```python
from build123d import *

# Parameters (mm, degrees)
F0_R     = 24
F0_R_2   = 21
F1_DEPTH = 17.5
F3_DEPTH = 12.5


with BuildPart() as f1:
    # F0 (on Front) → F1 (new body, symmetric)
    with BuildSketch(Plane.XZ):
        Circle(F0_R)
        Circle(F0_R_2, mode=Mode.SUBTRACT)
    extrude(amount=F1_DEPTH, both=True)

    # F2 (on Front) → F3 (join, symmetric)
    with BuildSketch(Plane.XZ):
        with BuildLine():
            Line((251.8847116829, -177.5), (236.7270928985, -165.6737260034))
            Line((236.7270928985, -165.6737260034), (28.1491312931, -2.9370746409))
            Line((28.1491312931, -2.9370746409), (23.9981043859, 0.3016386602))
            ThreePointArc((23.9981043859, 0.3016386602), (18.9220383946, -14.7633486375), (5.543918589, -23.350909333))
            Line((5.543918589, -23.350909333), (9.6949454961, -26.5896226342))
            Line((9.6949454961, -26.5896226342), (218.2729071015, -189.3262739966))
            Line((218.2729071015, -189.3262739966), (227.5, -196.5254343899))
            Line((227.5, -196.5254343899), (227.5, -222.5))
            Line((227.5, -222.5), (272.5, -222.5))
            Line((272.5, -222.5), (272.5, -177.5))
            Line((272.5, -177.5), (251.8847116829, -177.5))
        make_face()
        with BuildLine():
            Line((-272.5, -222.5), (-227.5, -222.5))
            Line((-227.5, -222.5), (-227.5, -196.5254343899))
            Line((-227.5, -196.5254343899), (-218.2729071015, -189.3262739966))
            Line((-218.2729071015, -189.3262739966), (-9.6949454961, -26.5896226342))
            Line((-9.6949454961, -26.5896226342), (-5.543918589, -23.350909333))
            ThreePointArc((-5.543918589, -23.350909333), (-18.9220383946, -14.7633486375), (-23.9981043859, 0.3016386602))
            Line((-23.9981043859, 0.3016386602), (-28.1491312931, -2.9370746409))
            Line((-28.1491312931, -2.9370746409), (-236.7270928985, -165.6737260034))
            Line((-236.7270928985, -165.6737260034), (-251.8847116829, -177.5))
            Line((-251.8847116829, -177.5), (-272.5, -177.5))
            Line((-272.5, -177.5), (-272.5, -222.5))
        make_face()
    extrude(amount=F3_DEPTH, both=True)


solid = f1.part
```
Read the model definition and answer for the solid it produces. Units are mm, in the model's axes. A direction names the side the tool comes from. Round coordinates to 2 decimals unless told otherwise and drop trailing zeros. Loops run counter-clockwise (first coordinate to the right, second up) from the corner with the lowest first, then second, coordinate; pieces in that order, holes last. Notation, with made-up numbers: (70.5, 74.5) -> (91.5, 74.5) arc R18 cw to (91.5, 84.5) -> close; hole circle Ø5 at (-37.5, 56). An arc over 180 degrees is marked (long way). One line per item, written item: value.
1) The mould has two halves that part along X. Classify faces 6 (the face through (-227.5, 0, -210)), 7 (the face through (272.5, 0, -200)), 8 (the face through (-0.1, -17.5, -21.2)): pulls with the +X half, pulls with the -X half, needs draft (parallel to the pull), parting line crosses it, or undercut.
Answer list:
face 6: undercut
face 7: pulls with the +X half
face 8: needs draft
2) A cutting plane is placed at C-C (z = -170). Determine the outline of the cut face in (x, y).
Answer list:
outline: (-242.27, -12.5) -> (-193.5, -12.5) -> (-193.5, 12.5) -> (-242.27, 12.5) -> close; (193.5, -12.5) -> (242.27, -12.5) -> (242.27, 12.5) -> (193.5, 12.5) -> close
3) A cutting plane is placed at B-B (y = 0). Determine the outline of the cut face in (x, z).
Answer list:
outline: (-272.5, -222.5) -> (-227.5, -222.5) -> (-227.5, -196.53) -> (-5.54, -23.35) arc R24 ccw to (5.54, -23.35) -> (227.5, -196.53) -> (227.5, -222.5) -> (272.5, -222.5) -> (272.5, -177.5) -> (251.88, -177.5) -> (24, 0.3) arc R24 ccw to (-24, 0.3) -> (-251.88, -177.5) -> (-272.5, -177.5) -> close; hole circle Ø42 at (0, 0)
4) A cutting plane is placed at D-D (x = 169). Determine the outline of the cut face in (y, z), and give its area (3 significant figures).
Answer list:
outline: (-12.5, -150.88) -> (12.5, -150.88) -> (12.5, -112.83) -> (-12.5, -112.83) -> close
area: 951 mm²
5) A cutting plane is placed at A-A (x = 0). Determine the outline of the cut face in (y, z), and give its area (3 significant figures).
Answer list:
outline: (-17.5, -24) -> (17.5, -24) -> (17.5, -21) -> (-17.5, -21) -> close; (-17.5, 21) -> (17.5, 21) -> (17.5, 24) -> (-17.5, 24) -> close
area: 210 mm²
6) For faces 1 (the face through (-262, 0, -177.5)), 2 (the face through (262, 0, -177.5)), 3 (the face through (20.03, 0.25, 6.31)), 4 (the face through (227.5, 0, -209)), 5 (the face through (250, 0, -222.5)), determine the directions among +Z, -Z, +X, -X, +Y, -Y from which every point of the face is accessible in a straight line to the end or side of a thin tool.
Answer list:
face 1: +Z, -X, +Y, -Y
face 2: +Z, +X, +Y, -Y
face 3: +Y, -Y
face 4: -Z, +Y, -Y
face 5: -Z, +X, -X, +Y, -Y
7) Consider L1, parallel to Z at x = 0, y = -9.5; L2, parallel to X at y = -11, z = -203.5; L3, parallel to X at y = 1, z = -49.5. Determine where each line is inside the solid, lowest interval first. Write a range as [from, to].
Answer list:
L1: z = [-24, -21], [21, 24]
L2: x = [-272.5, -227.5], [227.5, 272.5]
L3: x = [-87.83, -39.06], [39.06, 87.83]
8) Flat-ended cylindrical pins translate along their axes: P1, Ø5, axis at x = 24, y = 6.5, coming from the +Z side; P2, Ø10.5, axis at x = -267, y = -1.5, coming from the +Z side; P3, Ø3, axis at x = -108, z = -101.5, coming from the -Y side. Find the tip coordinate at first contact, or state that the pin passes through.
Answer list:
P1: stops at z = 10.67
P2: stops at z = -177.5
P3: stops at y = -12.5
